The model under review builds one solid part; all positions refer to its coordinate system, in mm. A direction names the side the tool comes from. Give positions to 0.01 mm unless a question says otherwise; leave off trailing zeros. Order: outer loops, then holes, each group sorted by start corner. A loop starts at its lowest first (then second) coordinate and runs counter-clockwise, first axis right, second up.
```python
from build123d import *

# Parameters (mm, degrees)
F0_W     = 300
F0_H     = 300
F0_W_2   = 2.5421465495
F0_H_2   = 11.9866538541
F0_R     = 40
F0_R_2   = 2
F1_DEPTH = 10
F2_SIZE  = 3


with BuildPart() as f1:
    # F0 (on Front) → F1 (new body)
    with BuildSketch(Plane.XZ):
        with Locations((-11.0126920044, -10.4479454458)):
            Rectangle(F0_W, F0_H)
        with BuildLine():
            Line((-110.3819430217, -143.5288141009), (-111.7330322611, -143.5288141009))
            Line((-111.7330322611, -143.5288141009), (-111.7330322611, -148.1277644634))
            Line((-111.7330322611, -148.1277644634), (-114.2751788106, -148.1277644634))
            Line((-114.2751788106, -148.1277644634), (-114.2751788106, -136.1411106094))
            Line((-114.2751788106, -136.1411106094), (-110.7833345822, -136.1411106094))
            add(Edge.make_bspline(
                [(-110.7833345822, -136.1411106094), (-108.33825658, -136.1411106094), (-107.1668753268, -137.0304683805)],
                knots=[0, 0, 0, 1, 1, 1], degree=2))
            add(Edge.make_bspline(
                [(-107.1668753268, -137.0304683805), (-105.9954940736, -137.9198261517), (-105.9954940736, -139.7326468594)],
                knots=[0, 0, 0, 1, 1, 1], degree=2))
            add(Edge.make_bspline(
                [(-105.9954940736, -139.7326468594), (-105.9954940736, -140.7899069826), (-106.5765936202, -141.6136778975)],
                knots=[0, 0, 0, 1, 1, 1], degree=2))
            add(Edge.make_bspline(
                [(-106.5765936202, -141.6136778975), (-107.1576931669, -142.4374488124), (-108.2254471872, -142.9044272291)],
                knots=[0, 0, 0, 1, 1, 1], degree=2))
            add(Edge.make_bspline(
                [(-108.2254471872, -142.9044272291), (-105.5180217599, -146.9472010504), (-104.6994977935, -148.1277644634)],
                knots=[0, 0, 0, 1, 1, 1], degree=2))
            Line((-104.6994977935, -148.1277644634), (-107.5197326136, -148.1277644634))
            Line((-107.5197326136, -148.1277644634), (-110.3819430217, -143.5288141009))
        make_face(mode=Mode.SUBTRACT)
        with Locations((-101.9199268242, -142.1344375364)):
            Rectangle(F0_W_2, F0_H_2, mode=Mode.SUBTRACT)
        with BuildLine():
            Line((-93.0827538088, -143.5130732554), (-93.0827538088, -141.3959295347))
            Line((-93.0827538088, -141.3959295347), (-88.3263949913, -141.3959295347))
            Line((-88.3263949913, -141.3959295347), (-88.3263949913, -147.6109400359))
            add(Edge.make_bspline(
                [(-88.3263949913, -147.6109400359), (-89.4833471361, -147.9887203281), (-90.5038786198, -148.1408818347)],
                knots=[0, 0, 0, 1, 1, 1], degree=2))
            add(Edge.make_bspline(
                [(-90.5038786198, -148.1408818347), (-91.5244101036, -148.2930433413), (-92.5895406496, -148.2930433413)],
                knots=[0, 0, 0, 1, 1, 1], degree=2))
            add(Edge.make_bspline(
                [(-92.5895406496, -148.2930433413), (-95.3022130254, -148.2930433413), (-96.7333182295, -146.6979709965)],
                knots=[0, 0, 0, 1, 1, 1], degree=2))
            add(Edge.make_bspline(
                [(-96.7333182295, -146.6979709965), (-98.1644234335, -145.1028986517), (-98.1644234335, -142.1173849538)],
                knots=[0, 0, 0, 1, 1, 1], degree=2))
            add(Edge.make_bspline(
                [(-98.1644234335, -142.1173849538), (-98.1644234335, -139.2158224319), (-96.5037642325, -137.5932036074)],
                knots=[0, 0, 0, 1, 1, 1], degree=2))
            add(Edge.make_bspline(
                [(-96.5037642325, -137.5932036074), (-94.8431050314, -135.970584783), (-91.9021903958, -135.970584783)],
                knots=[0, 0, 0, 1, 1, 1], degree=2))
            add(Edge.make_bspline(
                [(-91.9021903958, -135.970584783), (-90.0552645229, -135.970584783), (-88.3421358368, -136.7077810476)],
                knots=[0, 0, 0, 1, 1, 1], degree=2))
            Line((-88.3421358368, -136.7077810476), (-89.1868945457, -138.7409735924))
            add(Edge.make_bspline(
                [(-89.1868945457, -138.7409735924), (-90.4986316713, -138.0851050296), (-91.9179312413, -138.0851050296)],
                knots=[0, 0, 0, 1, 1, 1], degree=2))
            add(Edge.make_bspline(
                [(-91.9179312413, -138.0851050296), (-93.5654730711, -138.0851050296), (-94.557146338, -139.1922111636)],
                knots=[0, 0, 0, 1, 1, 1], degree=2))
            add(Edge.make_bspline(
                [(-94.557146338, -139.1922111636), (-95.548819605, -140.2993172976), (-95.548819605, -142.1672309645)],
                knots=[0, 0, 0, 1, 1, 1], degree=2))
            add(Edge.make_bspline(
                [(-95.548819605, -142.1672309645), (-95.548819605, -144.1190958075), (-94.7499716955, -145.147497714)],
                knots=[0, 0, 0, 1, 1, 1], degree=2))
            add(Edge.make_bspline(
                [(-94.7499716955, -145.147497714), (-93.951123786, -146.1758996205), (-92.426885246, -146.1758996205)],
                knots=[0, 0, 0, 1, 1, 1], degree=2))
            add(Edge.make_bspline(
                [(-92.426885246, -146.1758996205), (-91.6293490736, -146.1758996205), (-90.8108251072, -146.0132442169)],
                knots=[0, 0, 0, 1, 1, 1], degree=2))
            Line((-90.8108251072, -146.0132442169), (-90.8108251072, -143.5130732554))
            Line((-90.8108251072, -143.5130732554), (-93.0827538088, -143.5130732554))
        make_face(mode=Mode.SUBTRACT)
        Polygon((-75.6523908834, -136.1411106094), (-75.6523908834, -148.1277644634), (-78.1866670101, -148.1277644634), (-78.1866670101, -142.9542732399), (-82.9325319307, -142.9542732399), (-82.9325319307, -148.1277644634), (-85.4746784801, -148.1277644634), (-85.4746784801, -136.1411106094), (-82.9325319307, -136.1411106094), (-82.9325319307, -140.8397529934), (-78.1866670101, -140.8397529934), (-78.1866670101, -136.1411106094), align=None, mode=Mode.SUBTRACT)
        Polygon((-68.0023399667, -138.2556308559), (-68.0023399667, -148.1277644634), (-70.5444865162, -148.1277644634), (-70.5444865162, -138.2556308559), (-73.800218062, -138.2556308559), (-73.800218062, -136.1411106094), (-64.7492318951, -136.1411106094), (-64.7492318951, -138.2556308559), align=None, mode=Mode.SUBTRACT)
        with Locations((55.9873079956, -85.4479454458)):
            Circle(F0_R, mode=Mode.SUBTRACT)
        with Locations((-94.0126920044, -10.4479454458)):
            Circle(F0_R, mode=Mode.SUBTRACT)
        with Locations((-132.8097879887, 59.5533102751)):
            Circle(F0_R_2, mode=Mode.SUBTRACT)
        with Locations((55.9873079956, 64.5520545542)):
            Circle(F0_R, mode=Mode.SUBTRACT)
    extrude(amount=F1_DEPTH)

    # F2
    f2_edges = [f1.edges().sort_by_distance(p)[0] for p in [
        (-134.809788, -10, 59.55331),
    ]]
    chamfer(f2_edges, length=F2_SIZE)


solid = f1.part
```
Item 1: Draft analysis for pull direction Z (two halves, no side actions). For faces 3 (the conical face through (-130.72, -7.19, 60.21)), 4 (the flat face through (-13, 0, -8)), 5 (the flat face through (-13, -5, 139.552)), 6 (the flat face through (-70.544, -5, -143)), state which applies: released by +Z, released by -Z, zero draft, split by the parting line, or undercut.
Values found:
face 3: undercut
face 4: zero draft
face 5: released by +Z
face 6: undercut
Item 2: For line 1 (Z direction, x = -70, y = -8.25); line 2 (Z direction, x = 73.5, y = -4.5); line 3 (X direction, y = -4.25, z = 6.5), list the stretches that pass through material, from the lowest coordinate up.
Values found:
line 1: z = -160.45 to -148.13, -136.14 to -42.44, 21.54 to 139.55
line 2: z = -160.45 to -121.41, -49.49 to 28.59, 100.51 to 139.55
line 3: x = -161.01 to -130.24, -57.78 to 138.99
Item 3: Take a section at A-A (z = 91.5). Give the boundary of the cut face in (x, y), and give its area (3 significant figures).
Values found:
outline: (-161.01, -10) - (26.43, -10) - (26.43, 0) - (-161.01, 0) - close; (85.55, -10) - (138.99, -10) - (138.99, 0) - (85.55, 0) - close
area: 2,410 mm2
Item 4: Take a section at C-C (x = -57.5). Give the boundary of the cut face in (y, z), and give its area (3 significant figures).
Values found:
outline: (-10, -160.45) - (0, -160.45) - (0, -26.78) - (-10, -26.78) - close; (-10, 5.89) - (0, 5.89) - (0, 139.55) - (-10, 139.55) - close
area: 2,670 mm2
Item 5: Take a section at D-D (y = -4). Give the number of separate pieces and of enclosed holes in the cut face, and give its area (3 significant figures).
Values found:
separate pieces: 1
enclosed holes: 9
area: 74,600 mm2
Item 6: Clearance check with a flat-ended pin moving along its axis: pin 1 Ø10 at (x, z) = (-105, -43) entering from -Y. State where the tip first meets the part, or that it passes through.
Values found:
pin 1: passes through
Item 7: Take a section at B-B (x = 25). Give the boundary of the cut face in (y, z).
Values found:
outline: (-10, -160.45) - (0, -160.45) - (0, -110.74) - (-10, -110.74) - close; (-10, -60.15) - (0, -60.15) - (0, 39.26) - (-10, 39.26) - close; (-10, 89.85) - (0, 89.85) - (0, 139.55) - (-10, 139.55) - close
Item 8: For faces 1 (the flat face through (-103.191, -5, -142)), 2 (the flat face through (138.987, -5, -13)), list the 3-axis set-ups (+Z, -Z, +X, -X, +Y, -Y) from which the entire face can be reached by the end or side of a thin tool; tool diameter is ignored.
Values found:
face 1: +Y, -Y
face 2: +Z, -Z, +X, +Y, -Y
